Answer from the drawing. Dimensions are ordinates in mm from the lowest x, y and z of the part. A direction names the side the tool comes from. Round coordinates to 2 decimals unless told otherwise and drop trailing zeros. Write each loop counter-clockwise with the first axis right and the second up, starting at its lowest first coordinate (ties: lowest second). Pieces come first, ordered by that corner, then holes. Notation, with made-up numbers: (37, 83) - (43, 83) arc R21 ccw to (43, 98) - close; hole circle Ø9 at (1, 89.5). An arc over 180 degrees is marked (long way). Answer as a JSON object with one key per item and string values.
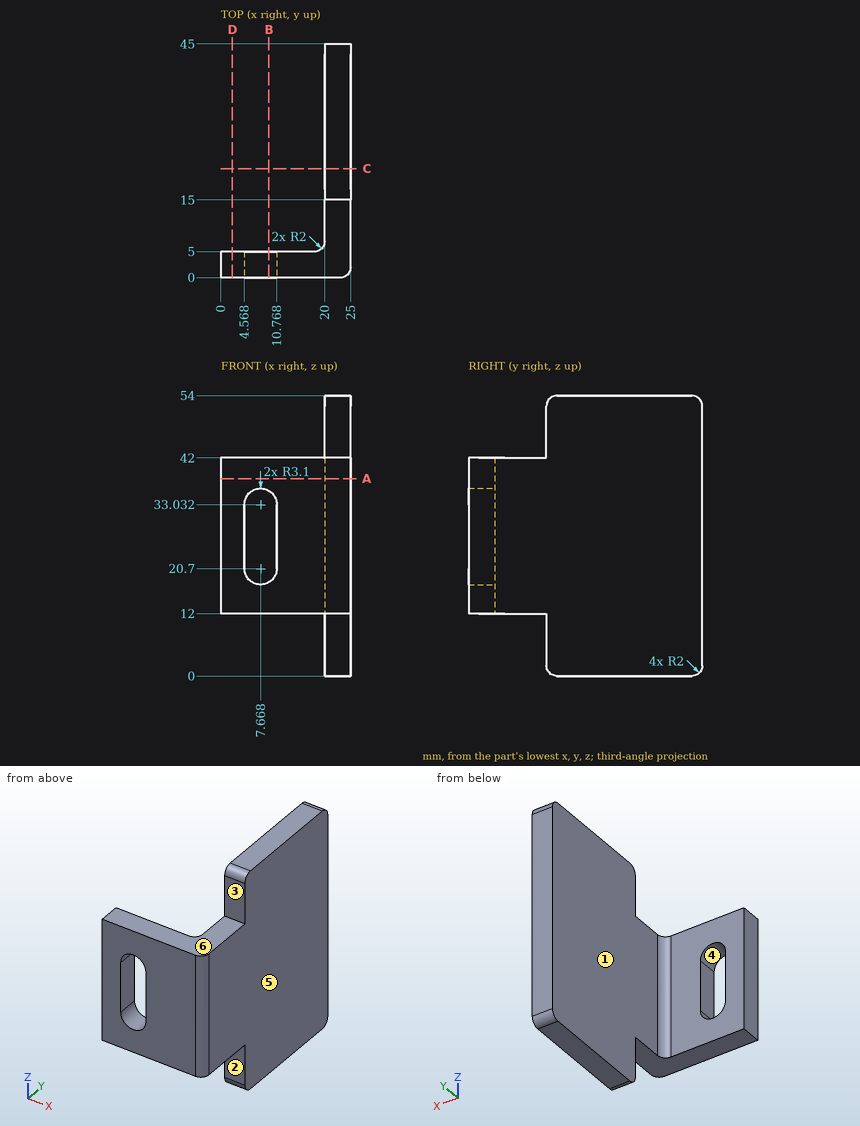
Item 1: A cutting plane is placed at D-D (x = 2.25). Write down the section's boundary in (y, z).
Results found:
{"outline": "(0, 12) - (5, 12) - (5, 42) - (0, 42) - close"}
Item 2: A cutting plane is placed at A-A (z = 38). Write down the section's boundary in (x, y).
Results found:
{"outline": "(0, 0) - (23, 0) arc R2 ccw to (25, 2) - (25, 45) - (20, 45) - (20, 7) arc R2 cw to (18, 5) - (0, 5) - close"}
Item 3: Determine the mould class of the marked faces 4, 5 and 6 for opening direction X: pulls with the +X half, pulls with the -X half, needs draft (parallel to the pull), parting line crosses it, or undercut.
Results found:
{"face 4": "undercut", "face 5": "pulls with the +X half", "face 6": "needs draft"}
Item 4: A cutting plane is placed at B-B (x = 9.25). Write down the section's boundary in (y, z).
Results found:
{"outline": "(0, 12) - (5, 12) - (5, 18.03) - (0, 18.03) - close; (0, 35.7) - (5, 35.7) - (5, 42) - (0, 42) - close"}
Item 5: For the marked faces 1, 2 and 3, determine the directions among +Z, -Z, +X, -X, +Y, -Y from which every point of the face is accessible in a straight line to the end or side of a thin tool.
Results found:
{"face 1": "+Z, -Z, -X, +Y", "face 2": "-Z, +X, -X, -Y", "face 3": "+Z, +X, -X, -Y"}
Item 6: Consider line 1 along X through (y, z) = (3, 20.5); line 2 along Y through (x, z) = (2.5, 38.5); line 3 along X through (y, z) = (41, 40). Determine where each line is inside the solid, lowest interval first.
Results found:
{"line 1": "0 to 4.57, 10.76 to 25", "line 2": "0 to 5", "line 3": "20 to 25"}
Item 7: A cutting plane is placed at C-C (y = 21). Write down the section's boundary in (x, z), and give its area (3 significant figures).
Results found:
{"outline": "(20, 0) - (25, 0) - (25, 54) - (20, 54) - close", "area": "270 mm²"}
Item 8: Each of these flat-tipped pins is pushed along its axis until it touches: P1, Ø10, axis at x = 4.5, y = 6.5, coming from the +Z side; P2, Ø1.5, axis at y = 31, z = 11.5, coming from the -X side; P3, Ø5.5, axis at x = 22, z = 8, coming from the -Y side. Where does it stop, or does it pass through?
Results found:
{"P1": "z = 42", "P2": "x = 20", "P3": "y = 15"}
